```python
from build123d import *

# Parameters (mm, degrees)
SZKIC1_W                                          = 31.8
SZKIC1_H                                          = 8.8
DODANIE_WYCI_GNI_CIE1_DEPTH                       = 8.75
SZKIC2_W                                          = 7.15
SZKIC2_H                                          = 17.5
WYTNIJ_WYCI_GNI_CIE1_DEPTH                        = 0.8
SZKIC3_W                                          = 7.15
SZKIC3_H                                          = 4
WYTNIJ_WYCI_GNI_CIE2_DEPTH                        = 26.228951623
POG_BIENIE_WALCOWE_POD_M2_5_RUB_Z_BEM_D           = 3.1
POG_BIENIE_WALCOWE_POD_M2_5_RUB_Z_BEM_CBORE_D     = 5.5
POG_BIENIE_WALCOWE_POD_M2_5_RUB_Z_BEM_CBORE_DEPTH = 2.5
SZKIC6_R                                          = 5
WYTNIJ_WYCI_GNI_CIE3_DEPTH                        = 26.228951623


with BuildPart() as part:
    # Szkic1 → Dodanie-wyciągnięcie1 (new, symmetric)
    with BuildSketch(Plane.XY):
        with Locations((0, 4.4)):
            Rectangle(SZKIC1_W, SZKIC1_H)
    extrude(amount=DODANIE_WYCI_GNI_CIE1_DEPTH, both=True)

    # Szkic2 → Wytnij-wyciągnięcie1 (cut)
    with BuildSketch(Plane.XZ):
        with Locations((12.325, 0)):
            Rectangle(SZKIC2_W, SZKIC2_H)
    wytnij_wyci_gni_cie1 = extrude(amount=-WYTNIJ_WYCI_GNI_CIE1_DEPTH, mode=Mode.SUBTRACT)

    # Szkic3 → Wytnij-wyciągnięcie2 (cut, through all)
    with BuildSketch(Plane.XY.offset(8.75)):
        with Locations((12.325, 6.8)):
            Rectangle(SZKIC3_W, SZKIC3_H)
    wytnij_wyci_gni_cie2 = extrude(amount=-WYTNIJ_WYCI_GNI_CIE2_DEPTH, mode=Mode.SUBTRACT)

    # Pogłębienie walcowe pod M2.5 Śrubę z łbem walcowym z gniazdem1 (through all)
    with Locations(Plane(origin=(0, 4.8, 0), x_dir=(1, 0, 0), z_dir=(0, 1, 0))):
        with Locations((12.5, 5.5), (12.5, -5.5)):
            pog_bienie_walcowe_pod_m2_5_rub_z_bem = CounterBoreHole(POG_BIENIE_WALCOWE_POD_M2_5_RUB_Z_BEM_D / 2, POG_BIENIE_WALCOWE_POD_M2_5_RUB_Z_BEM_CBORE_D / 2, POG_BIENIE_WALCOWE_POD_M2_5_RUB_Z_BEM_CBORE_DEPTH)

    # Lustro1: Wytnij-wyciągnięcie1, Wytnij-wyciągnięcie2, Pogłębienie walcowe pod M2.5 Śrubę z łbem walcowym z gniazdem1 across plane
    add(wytnij_wyci_gni_cie1.mirror(Plane(origin=(0, 0, 0), x_dir=(0, 0, 1), z_dir=(1, 0, 0))), mode=Mode.SUBTRACT)
    add(wytnij_wyci_gni_cie2.mirror(Plane(origin=(0, 0, 0), x_dir=(0, 0, 1), z_dir=(1, 0, 0))), mode=Mode.SUBTRACT)
    add(pog_bienie_walcowe_pod_m2_5_rub_z_bem.mirror(Plane(origin=(0, 0, 0), x_dir=(0, 0, 1), z_dir=(1, 0, 0))), mode=Mode.SUBTRACT)

    # Szkic6 → Wytnij-wyciągnięcie3 (cut, through all)
    with BuildSketch(Plane.XY.offset(8.75)):
        Circle(SZKIC6_R)
    extrude(amount=-WYTNIJ_WYCI_GNI_CIE3_DEPTH, mode=Mode.SUBTRACT)

    # Szkic7 → Wycięcie-obrót5 (revolve, cut)
    with BuildSketch(Plane.XY, mode=Mode.PRIVATE) as wyci_cie_obr_t5_sk:
        Polygon((0, 0), (0, 8.8), (2.770725942, 8.8), (0.75, 5.3), (0.75, 0), align=None)
    revolve(wyci_cie_obr_t5_sk.sketch.rotate(Axis((0, 0, 0), (0, 1, 0)), 90), axis=Axis((0, 0, 0), (0, 1, 0)), mode=Mode.SUBTRACT)


solid = part.part
```
Source: CAD feature listing. Evaluate the final solid. Frame: model axes, mm. A direction names the side the tool comes from. Coordinates: 2 decimals unless noted, no trailing zeros. Loops run counter-clockwise (first coordinate to the right, second up) from the corner with the lowest first, then second, coordinate; pieces in that order, holes last. Notation, with made-up numbers: M 33,41 L 62,41 A11 ccw 62,47 Z; hole C -39.5,65 d8. An arc over 180 degrees is marked long. Put each result on its own line as item: value. Start each with the question number.
1) Reachability of faces 1 (the face through (12, 0.8, 0)), 2 (the face through (-12, 4.8, 0)), 3 (the face through (-14, 2.3, -4)) from +Z, -Z, +X, -X, +Y, -Y: full face, straight path, thin tool, end or side. Return the list, or none.
2) Pull-direction query (X, two-part tool) for faces 4 (the face through (-8.75, 7, 0)), 5 (the face through (13.77, 3.57, 7.94)), 6 (the face through (-7, 0, 0)); classes: pulls with the +X half, pulls with the -X half, needs draft (parallel to the pull), parting line crosses it, or undercut.
3) Ray query, L1, parallel to Z at x = 12.5, y = 1.2; L2, parallel to Z at x = 12.5, y = 3.75; L3, parallel to X at y = 1, z = 6.25. Return the intervals inside material, ascending. Write a range as from..to.
4) Cut plane D-D on z = 5.5. Give the number of separate pieces and of enclosed holes in the cut face, then the cut area to 3 significant figures.
5) Contact query for flat-ended pins moving along their axis: pin 1 Ø5.5 at (x, z) = (-12.5, -4) entering from -Y; pin 2 Ø1.9 at (x, z) = (12.5, -5.5) entering from -Y; pin 3 Ø7 at (x, z) = (12.5, -5.5) entering from +Y; pin 4 Ø4 at (x, z) = (-10, -6) entering from +Y. Output: stop coordinate, or through.
6) Cut plane B-B on y = 4.5. Return the cut outline in (x, z), then the cut area to 3 significant figures.
7) Cut plane A-A on x = -12.5. Return the cut outline in (y, z).
8) Cut plane C-C on z = 0. Return the cut outline in (x, y), then the cut area to 3 significant figures.
The answers:
1. face 1: +Z, -Z, +X, -Y
1. face 2: +Z, -Z, -X, +Y
1. face 3: +Y
2. face 4: pulls with the -X half
2. face 5: undercut
2. face 6: needs draft
3. L1: z = -8.75..-7.05, -3.95..3.95, 7.05..8.75
3. L2: z = -8.75..-8.25, -2.75..2.75, 8.25..8.75
3. L3: x = -15.9..-13.86, -11.14..-4.9, 4.9..11.14, 13.86..15.9
4. separate pieces: 3
4. enclosed holes: 0
4. area: 135 mm²
5. pin 1: stops at y = 0.8
5. pin 2: passes through
5. pin 3: stops at y = 4.8
5. pin 4: stops at y = 8.8
6. outline: M -15.9,-8.75 L -2.18,-8.75 L -2.18,8.75 L -15.9,8.75 Z; M 2.18,-8.75 L 15.9,-8.75 L 15.9,8.75 L 2.18,8.75 Z; hole C -12.5,-5.5 d5.5; hole C -12.5,5.5 d5.5; hole C 12.5,-5.5 d5.5; hole C 12.5,5.5 d5.5
6. area: 385 mm²
7. outline: M 0.8,-8.75 L 4.8,-8.75 L 4.8,-8.25 L 2.3,-8.25 L 2.3,-7.05 L 0.8,-7.05 Z; M 0.8,-3.95 L 2.3,-3.95 L 2.3,-2.75 L 4.8,-2.75 L 4.8,2.75 L 2.3,2.75 L 2.3,3.95 L 0.8,3.95 Z; M 0.8,7.05 L 2.3,7.05 L 2.3,8.25 L 4.8,8.25 L 4.8,8.75 L 0.8,8.75 Z
8. outline: M -15.9,0.8 L -8.75,0.8 L -8.75,0 L -5,0 A5 cw -0.75,4.94 L -0.75,5.3 L -2.77,8.8 L -8.75,8.8 L -8.75,4.8 L -15.9,4.8 Z; M 0.75,4.94 A5 cw 5,0 L 8.75,0 L 8.75,0.8 L 15.9,0.8 L 15.9,4.8 L 8.75,4.8 L 8.75,8.8 L 2.77,8.8 L 0.75,5.3 Z
8. area: 159 mm²
